Work out the finished part from the listing and answer in its coordinate system (mm). Face numbers are marked on the shaded views. A direction names the side the tool comes from. Round coordinates to 2 decimals unless told otherwise and drop trailing zeros. Loops run counter-clockwise (first coordinate to the right, second up) from the corner with the lowest first, then second, coordinate; pieces in that order, holes last. Notation, with made-up numbers: (7, 23.5) - (63, 23.5) arc R13 ccw to (63, 33.5) - close; hole circle Ø5 at (33.5, 65.5). An arc over 180 degrees is marked (long way). Return JSON: item names as keys, results as strings.
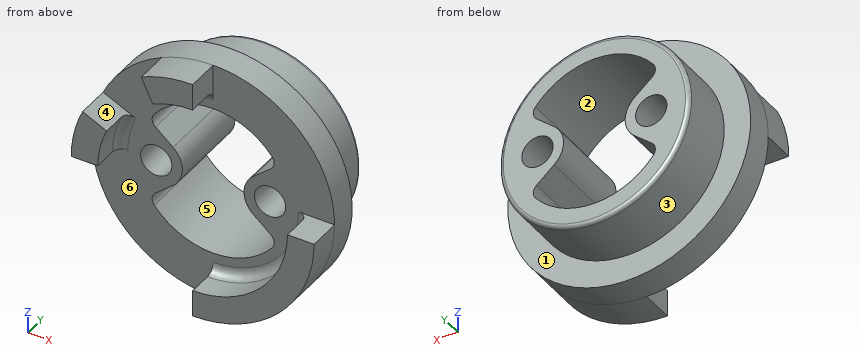
from build123d import *
from build123d.topology import SkipClean

# Parameters (mm, degrees)
SKETCH_1_R             = 12.8
EXTRUDE_1_DEPTH        = 3
SKETCH_2_R             = 10.01
EXTRUDE_2_DEPTH        = 5.95
SKETCH_3_R             = 8
CUT_EXTRUDE_1_DEPTH    = 21.193625232
EXTRUDE_START          = 8.95
SKETCH_4_R             = 1.65
EXTRUDE_3_DEPTH        = 8.95
FILLET_1_R             = 1
FILLET_1_OF_MIRROR_1_R = 1
FILLET_2_R             = 0.4
EXTRUDE_START_2        = 3.5
EXTRUDE_4_DEPTH        = 3.5
FILLET_3_R             = 1


with BuildPart() as part:
    # 草图1 → 凸台-拉伸1 (new body)
    with BuildSketch(Plane(origin=(0, 0, 0), x_dir=(1, 0, 0), z_dir=(0, 1, 0))):
        with Locations(Location((0, 0, 0), (0, 0, 270))):
            Circle(SKETCH_1_R)
    extrude(amount=EXTRUDE_1_DEPTH)

    # 草图2 → 凸台-拉伸2 (add)
    with BuildSketch(Plane(origin=(0, 3, 0), x_dir=(1, 0, 0), z_dir=(0, 1, 0))):
        with Locations(Location((0, 0, 0), (0, 0, 270))):
            Circle(SKETCH_2_R)
    extrude(amount=EXTRUDE_2_DEPTH)

    # 草图3 → 切除-拉伸1 (cut, through all)
    with BuildSketch(Plane(origin=(0, 8.95, 0), x_dir=(1, 0, 0), z_dir=(0, 1, 0))):
        with Locations(Location((0, 0, 0), (0, 0, 270))):
            Circle(SKETCH_3_R)
    extrude(amount=-CUT_EXTRUDE_1_DEPTH, mode=Mode.SUBTRACT)

    # 草图4 → 凸台-拉伸3 (add)
    with BuildSketch(Plane(origin=(0, 0, 0), x_dir=(1, 0, 0), z_dir=(0, 1, 0)).offset(EXTRUDE_START)):
        with BuildLine():
            Line((-6.780819092, 4.245055058), (-4.232334073, 2.106622219))
            ThreePointArc((-4.232334073, 2.106622219), (-3.25, 0), (-4.232334073, -2.106622219))
            Line((-4.232334073, -2.106622219), (-6.780819092, -4.245055058))
            ThreePointArc((-6.780819092, -4.245055058), (-8, 0), (-6.780819092, 4.245055058))
        make_face()
        with Locations(Location((-6, 0, 0), (0, 0, 270))):
            Circle(SKETCH_4_R, mode=Mode.SUBTRACT)
    extrude_3 = extrude(amount=-EXTRUDE_3_DEPTH)

    # 圆角1
    fillet_1_edges = [part.edges().sort_by_distance(p)[0] for p in [
        (-6.780819092, 4.475, 4.245055058),
        (-6.780819092, 4.475, -4.245055058),
    ]]
    fillet(fillet_1_edges, radius=FILLET_1_R)

    # 镜向1: 凸台-拉伸3 across plane
    add(extrude_3.mirror(Plane(origin=(0, 0, 0), x_dir=(0, 0, 1), z_dir=(1, 0, 0))))

    # 圆角1 of 镜向1
    fillet_1_of_mirror_1_edges = [part.edges().sort_by_distance(p)[0] for p in [
        (6.780819092, 4.475, 4.245055058),
        (6.780819092, 4.475, -4.245055058),
    ]]
    fillet(fillet_1_of_mirror_1_edges, radius=FILLET_1_OF_MIRROR_1_R)

    # 圆角2
    fillet_2_edges = [part.edges().sort_by_distance(p)[0] for p in [
        (0, 8.95, -10.01),
    ]]
    fillet(fillet_2_edges, radius=FILLET_2_R)

    # 草图5 → 凸台-拉伸4 (add)
    with SkipClean():  # the faces are left unmerged after this step: merging them gives an invalid solid
        with BuildSketch(Plane.XZ.offset(EXTRUDE_START_2)):
            with BuildLine():
                ThreePointArc((0.005, -12.799999023), (9.050966799, -9.050966799), (12.799999023, -0.005))
                Line((12.799999023, -0.005), (9.99999875, -0.005))
                ThreePointArc((9.99999875, -0.005), (7.071067812, -7.071067812), (0.005, -9.99999875))
                Line((0.005, -9.99999875), (0.005, -12.799999023))
            make_face()
            with BuildLine():
                Line((-9.06307787, 4.226182617), (-11.600739674, 5.40951375))
                ThreePointArc((-11.600739674, 5.40951375), (-12.496047554, 2.772867746), (-12.799999023, 0.005))
                Line((-12.799999023, 0.005), (-9.99999875, 0.005))
                ThreePointArc((-9.99999875, 0.005), (-9.762418667, 2.166836812), (-9.06307787, 4.226182617))
            make_face()
            with BuildLine():
                Line((-0.005, 9.99999875), (-0.005, 12.799999023))
                ThreePointArc((-0.005, 12.799999023), (-2.772867746, 12.496047554), (-5.40951375, 11.600739674))
                Line((-5.40951375, 11.600739674), (-4.226182617, 9.06307787))
                ThreePointArc((-4.226182617, 9.06307787), (-2.166836812, 9.762418667), (-0.005, 9.99999875))
            make_face()
        extrude(amount=-EXTRUDE_4_DEPTH)

    # 圆角3
    fillet_3_edges = [part.edges().sort_by_distance(p)[0] for p in [
        (-2.166836812, 0, 9.762418667),
        (7.071067812, 0, -7.071067812),
        (-9.762418667, 0, 2.166836812),
    ]]
    fillet(fillet_3_edges, radius=FILLET_3_R)


solid = part.part
1) Find the intervals of material crossed by L1, parallel to X at y = 3.5, z = 0; L2, parallel to X at y = 2, z = 0; L3, parallel to Z at x = 6, y = 2.25, in increasing order.
Verdict:
{"L1": "x = -10.01 to -7.65, -4.35 to -3.25, 3.25 to 4.35, 7.65 to 10.01", "L2": "x = -12.8 to -7.65, -4.35 to -3.25, 3.25 to 4.35, 7.65 to 12.8", "L3": "z = -11.31 to -5.29, -3.59 to -1.65, 1.65 to 3.59, 5.29 to 11.31"}
2) Determine the mould class of the marked faces 1, 2 and 3 for opening direction Z: pulls with the +Z half, pulls with the -Z half, needs draft (parallel to the pull), parting line crosses it, or undercut.
Verdict:
{"face 1": "needs draft", "face 2": "undercut", "face 3": "parting line crosses it"}
3) Section C-C (z = -0.75) is taken. Count the separate pieces of the cut face and the enclosed holes in it, and give its area (3 significant figures).
Verdict:
{"separate pieces": "4", "enclosed holes": "0", "area": "92.8 mm2"}
4) Flat-ended cylindrical pins translate along their axes: pin 1 (3 mm diameter, centred on y = -2, z = 11, fed in from +X) (3 decimals); pin 2 (5 mm diameter, centred on x = 7, z = 4, fed in from -Y); pin 3 (3 mm diameter, centred on x = -11, y = -2, fed in from -Z) (3 decimals). Find the tip coordinate at first contact, or state that the pin passes through.
Verdict:
{"pin 1": "stops at x = -0.005", "pin 2": "stops at y = 0", "pin 3": "stops at z = 0.005"}
5) A tool of negligible diameter and unlimited length cuts with its end or side. For the marked faces 4, 5 and 6, from which of +Z, -Z, +X, -X, +Y, -Y can it reach the whole face along a straight path? Write none if from no direction.
Verdict:
{"face 4": "+Z, +X, -Y", "face 5": "+Y, -Y", "face 6": "-Y"}
6) Section A-A (y = 5.25) is taken. Give the vertices of the cut face in (x, z), and give its area (3 significant figures).
Verdict:
{"outline": "circle Ø20.02 at (0, 0); hole circle Ø3.3 at (-6, 0); hole (-6.21, -5.05) arc R8 ccw to (6.21, -5.05) arc R1 ccw to (6.07, -3.65) - (4.23, -2.11) arc R2.75 cw to (4.23, 2.11) - (6.07, 3.65) arc R1 ccw to (6.21, 5.05) arc R8 ccw to (-6.21, 5.05) arc R1 ccw to (-6.07, 3.65) - (-4.23, 2.11) arc R2.75 cw to (-4.23, -2.11) - (-6.07, -3.65) arc R1 ccw to start; hole circle Ø3.3 at (6, 0)", "area": "150 mm2"}
7) Section B-B (y = 1.25) is taken. Give the vertices of the cut face in (x, z), and give its area (3 significant figures).
Verdict:
{"outline": "circle Ø25.6 at (0, 0); hole circle Ø3.3 at (-6, 0); hole (-6.21, -5.05) arc R8 ccw to (6.21, -5.05) arc R1 ccw to (6.07, -3.65) - (4.23, -2.11) arc R2.75 cw to (4.23, 2.11) - (6.07, 3.65) arc R1 ccw to (6.21, 5.05) arc R8 ccw to (-6.21, 5.05) arc R1 ccw to (-6.07, 3.65) - (-4.23, 2.11) arc R2.75 cw to (-4.23, -2.11) - (-6.07, -3.65) arc R1 ccw to start; hole circle Ø3.3 at (6, 0)", "area": "349 mm2"}
